Verification items for the finished model (mm, model axes). A direction names the side the tool comes from. Give positions to 0.01 mm unless a question says otherwise; leave off trailing zeros.
from build123d import *

# Parameters (mm, degrees)
SKETCH1_W           = 73
SKETCH1_H           = 34.5
BOSS_EXTRUDE1_DEPTH = 34.5
CUT_EXTRUDE1_DEPTH  = 0.5
CUT_EXTRUDE2_START  = -0.5
CUT_EXTRUDE2_DEPTH  = 0.5
FILLET1_R           = 2
FILLET2_R           = 1


with BuildPart() as part:
    # Sketch1 → Boss-Extrude1 (new body)
    with BuildSketch(Plane(origin=(0, 0, -15), x_dir=(-1, 0, 0), z_dir=(0, 0, -1))):
        with Locations((-32.5, -4.75)):
            Rectangle(SKETCH1_W, SKETCH1_H)
    extrude(amount=-BOSS_EXTRUDE1_DEPTH)

    # Sketch2 → Cut-Extrude1 (cut)
    with BuildSketch(Plane(origin=(69, 0, 0), x_dir=(0, 0, -1), z_dir=(1, 0, 0))):
        with BuildLine():
            Line((-15.375, 0.375), (-15.375, -9.875))
            ThreePointArc((-15.375, -9.875), (-13.031854249, -15.531854249), (-7.375, -17.875))
            Line((-7.375, -17.875), (2.875, -17.875))
            ThreePointArc((2.875, -17.875), (8.531854249, -15.531854249), (10.875, -9.875))
            Line((10.875, -9.875), (10.875, 0.375))
            ThreePointArc((10.875, 0.375), (8.531854249, 6.031854249), (2.875, 8.375))
            Line((2.875, 8.375), (-7.375, 8.375))
            ThreePointArc((-7.375, 8.375), (-13.031854249, 6.031854249), (-15.375, 0.375))
        make_face()
    extrude(amount=-CUT_EXTRUDE1_DEPTH, mode=Mode.SUBTRACT)

    # Sketch3 → Cut-Extrude2 (cut)
    with BuildSketch(Plane.ZY.offset(4).offset(CUT_EXTRUDE2_START)):
        with BuildLine():
            Line((7.375, 8.375), (-2.875, 8.375))
            ThreePointArc((-2.875, 8.375), (-8.531854249, 6.031854249), (-10.875, 0.375))
            Line((-10.875, 0.375), (-10.875, -9.875))
            ThreePointArc((-10.875, -9.875), (-8.531854249, -15.531854249), (-2.875, -17.875))
            Line((-2.875, -17.875), (7.375, -17.875))
            ThreePointArc((7.375, -17.875), (13.031854249, -15.531854249), (15.375, -9.875))
            Line((15.375, -9.875), (15.375, 0.375))
            ThreePointArc((15.375, 0.375), (13.031854249, 6.031854249), (7.375, 8.375))
        make_face()
    extrude(amount=CUT_EXTRUDE2_DEPTH, mode=Mode.SUBTRACT)

    # Fillet1
    fillet1_edges = [part.edges().sort_by_distance(p)[0] for p in [
        (-4, -4.75, 19.5),
        (69, -4.75, 19.5),
        (-4, -4.75, -15),
        (69, -4.75, -15),
    ]]
    fillet(fillet1_edges, radius=FILLET1_R)

    # Fillet2
    fillet2_edges = [part.edges().sort_by_distance(p)[0] for p in [
        (32.5, -22, -15),
        (32.5, 12.5, -15),
        (-4, 12.5, 2.25),
        (32.5, 12.5, 19.5),
        (69, 12.5, 2.25),
        (68.414213562, 12.5, 18.914213562),
        (68.414213562, 12.5, -14.414213562),
        (-3.414213562, 12.5, 18.914213562),
        (-3.414213562, 12.5, -14.414213562),
        (-4, -22, 2.25),
        (69, -22, 2.25),
        (32.5, -22, 19.5),
        (68.414213562, -22, 18.914213562),
        (68.414213562, -22, -14.414213562),
        (-3.414213562, -22, 18.914213562),
        (-3.414213562, -22, -14.414213562),
    ]]
    fillet(fillet2_edges, radius=FILLET2_R)


solid = part.part
(1) Go/stop test with flat-tipped pins: pin 1 (8 mm diameter, centred on y = -12.5, z = 6.5, fed in from -X); pin 2 (0.6 mm diameter, centred on x = 68.5, z = 0, fed in from -Y); pin 3 (0.6 mm diameter, centred on x = 69, z = 3, fed in from +Y). Record where each tip stops, or that it passes through.
Solved:
pin 1: stops at x = -3.5
pin 2: stops at y = -21.98
pin 3: stops at y = 12.21
(2) Release check for a two-part mould opening along Z. For faces 1 (the flat face through (33, -5, -15)), 2 (the cylindrical face through (68.754, 5.969, -8.594)), 3 (the flat face through (33, -5, 19.5)) record: pulls with the +Z half, pulls with the -Z half, needs draft (parallel to the pull), parting line crosses it, or undercut.
Solved:
face 1: pulls with the -Z half
face 2: undercut
face 3: pulls with the +Z half
(3) Scan line: line 1 (X direction, y = -14, z = 0). Record every from-to range of solid material in increasing order.
Solved:
line 1: x = -3.5 to 68.5
(4) Set-up check for faces 4 (the flat face through (33, -22, 2)), 5 (the cylindrical face through (-3.746, 6.094, -8.469)), 6 (the cylindrical face through (68.754, 6.094, 12.969)): record each of +Z, -Z, +X, -X, +Y, -Y from which the full face is reachable in a straight line by a thin tool's end or side.
Solved:
face 4: +Z, -Z, +X, -X, -Y
face 5: -X
face 6: +X
